Work out the finished part from the listing and answer in its coordinate system (mm). Round coordinates to 2 decimals unless told otherwise and drop trailing zeros. Write each loop counter-clockwise with the first axis right and the second up, starting at its lowest first coordinate (ties: lowest second). Pieces come first, ordered by that corner, then holes. Notation, with made-up numbers: (60.5, 27.5) - (76.5, 27.5) arc R9 ccw to (76.5, 40.5) - close; hole circle Ø4 at (50, 17). An arc over 180 degrees is marked (long way). Answer as a JSON object with one key per item and string values.
```python
from build123d import *

# Parameters (mm, degrees)
SKETCH2_R           = 2
BOSS_EXTRUDE1_DEPTH = 2.5
FILLET1_R           = 1


with BuildPart() as part:
    # Sketch1 → Revolve1 (revolve)
    with BuildSketch(Plane(origin=(0, 0, 0), x_dir=(1, 0, 0), z_dir=(0, 1, 0))):
        with BuildLine():
            Line((25, 0), (-25, 0))
            ThreePointArc((-25, 0), (0, -25), (25, 0))
        make_face()
    revolve(axis=Axis((25, 0, 0), (-1, 0, 0)))

    # Sketch2 → Boss-Extrude1 (add, symmetric)
    with BuildSketch(Plane.XY):
        with BuildLine():
            Line((-3.7, 30), (-3.7, 20))
            Line((-3.7, 20), (3.7, 20))
            Line((3.7, 20), (3.7, 30))
            ThreePointArc((3.7, 30), (0, 33.7), (-3.7, 30))
        make_face()
        with Locations((0, 30)):
            Circle(SKETCH2_R, mode=Mode.SUBTRACT)
    extrude(amount=BOSS_EXTRUDE1_DEPTH, both=True)

    # Fillet1
    fillet1_edges = [part.edges().sort_by_distance(p)[0] for p in [
        (0, 33.7, -2.5),
        (3.7, 27.298983698, -2.5),
        (-3.7, 27.298983698, -2.5),
    ]]
    fillet(fillet1_edges, radius=FILLET1_R)
    fillet1_2_edges = [part.edges().sort_by_distance(p)[0] for p in [
        (3.7, 27.298983698, 2.5),
        (0, 33.7, 2.5),
        (-3.7, 27.298983698, 2.5),
    ]]
    fillet(fillet1_2_edges, radius=FILLET1_R)
    fillet1_3_edges = [part.edges().sort_by_distance(p)[0] for p in [
        (0, 24.874685928, -2.5),
    ]]
    fillet(fillet1_3_edges, radius=FILLET1_R)
    # the kernel refuses this fillet: 1 mm, written as the material it takes off along each edge
    with BuildSketch(Plane(origin=(0, 30, -2.5), x_dir=(1, 0, 0), z_dir=(0, -1, 0))) as fillet1_4_piece_1:
        with BuildLine():
            CenterArc((2 + FILLET1_R, FILLET1_R), FILLET1_R, 180, 90)
            Line((2, FILLET1_R), (2 - FILLET1_R * 0.02, FILLET1_R))
            Line((2 - FILLET1_R * 0.02, FILLET1_R), (2 - FILLET1_R * 0.02, -FILLET1_R * 0.02))
            Line((2 - FILLET1_R * 0.02, -FILLET1_R * 0.02), (2 + FILLET1_R, -FILLET1_R * 0.02))
            Line((2 + FILLET1_R, -FILLET1_R * 0.02), (2 + FILLET1_R, 0))
        make_face()
    revolve(axis=Axis((0, 30, -2.5), (0, 0, 1)), mode=Mode.SUBTRACT)
    # the kernel refuses this fillet: 1 mm, written as the material it takes off along each edge
    with BuildSketch(Plane(origin=(0, 30, 2.5), x_dir=(1, 0, 0), z_dir=(0, -1, 0))) as fillet1_5_piece_1:
        with BuildLine():
            CenterArc((2 + FILLET1_R, -FILLET1_R), FILLET1_R, 90, 90)
            Line((2, -FILLET1_R), (2 - FILLET1_R * 0.02, -FILLET1_R))
            Line((2 - FILLET1_R * 0.02, -FILLET1_R), (2 - FILLET1_R * 0.02, FILLET1_R * 0.02))
            Line((2 - FILLET1_R * 0.02, FILLET1_R * 0.02), (2 + FILLET1_R, FILLET1_R * 0.02))
            Line((2 + FILLET1_R, FILLET1_R * 0.02), (2 + FILLET1_R, 0))
        make_face()
    revolve(axis=Axis((0, 30, 2.5), (0, 0, 1)), mode=Mode.SUBTRACT)


solid = part.part
```
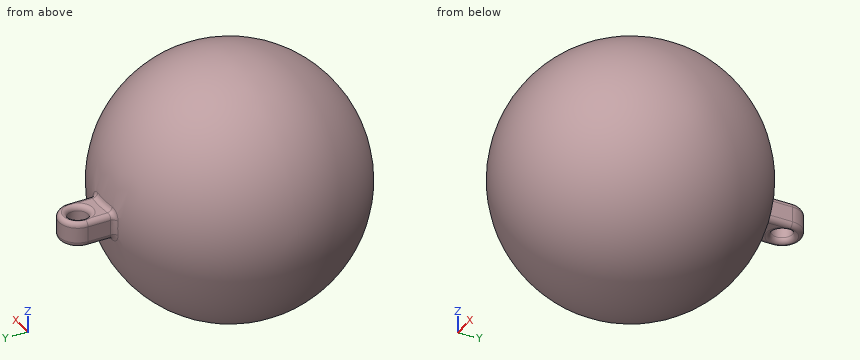
Item 1: A cutting plane is placed at A-A (y = 22.5). Write down the section's boundary in (x, z), and give its area (3 significant figures).
Results found:
{"outline": "circle Ø21.79 at (0, 0)", "area": "373 mm²"}
Item 2: Consider line 1 along Y through (x, z) = (0, 0); line 2 along Z through (x, y) = (-18, 15); line 3 along Y through (x, z) = (17, -15.5). Determine where each line is inside the solid, lowest interval first.
Results found:
{"line 1": "-25 to 28, 32 to 33.7", "line 2": "-8.72 to 8.72", "line 3": "-9.79 to 9.79"}
Item 3: Each of these flat-tipped pins is pushed along its axis until it touches: P1, Ø2, axis at y = 13, z = -19, coming from the -X side; P2, Ø2.5, axis at y = 28.5, z = 0.5, coming from the +X side; P3, Ø0.9, axis at x = -1, y = 27.5, coming from the +Z side. Where does it stop, or does it pass through?
Results found:
{"P1": "x = -11.83", "P2": "x = 3.7", "P3": "z = 2.5"}
Item 4: A cutting plane is placed at B-B (x = -5.5). Write down the section's boundary in (y, z) (1 decimal), and give its area (3 significant figures).
Results found:
{"outline": "circle Ø48.8 at (0, 0)", "area": "1,870 mm²"}
